Work out the finished part from the listing and answer in its coordinate system (mm). A direction names the side the tool comes from. Coordinates: 2 decimals unless noted, no trailing zeros. Loops run counter-clockwise (first coordinate to the right, second up) from the corner with the lowest first, then second, coordinate; pieces in that order, holes last. Notation, with made-up numbers: M -37.75,61 L -15.75,61 A4 ccw -15.75,66 Z; hole C 13,-35.5 d7. An arc over 180 degrees is marked long. Write each question's results on one line, items separated by ' | '.
Autodesk Fusion 360 part; units mm, degrees
sketch "Sketch1" plane through (0, 0, 0) normal (0, 0, 1) x (1, 0, 0)
  line L0 (0, 0) -> (139.7, 0)
  line L1 (139.7, 0) -> (139.7, 25)
  line L2 (139.7, 25) -> (0, 25)
  line L3 (0, 25) -> (0, 0)
  dimension "d1" = 139.7
  dimension "d2" = 25
extrude "Extrude1" add sketch "Sketch1" along normal blind 5
sketch "Sketch2" plane through (0, 0, 0) normal (0, 0, 1) x (1, 0, 0)
  point P0 (6.35, 12.5)
  point P1 (133.35, 12.5)
hole "Hole1" at (6.35, 12.5, 0) at (133.35, 12.5, 0) direction (0, 0, 1) diameter 5.5 depth 13 tip angle 118 counterbore diameter 9.1 counterbore depth 1
sketch "Sketch4" plane through (0, 0, 0) normal (0, 0, -1) x (1, 0, 0)
  circle A0 centre (6.35, -12.5) radius 4.55
  circle A1 centre (133.35, -12.5) radius 4.55
  line L0 (0, 0) -> (0, -25)
  line L1 (0, -25) -> (139.7, -25)
  line L2 (139.7, -25) -> (139.7, 0)
  line L3 (139.7, 0) -> (0, 0)
  point P0 (49.85, -12.5)
  point P1 (89.85, -12.5)
hole "Hole3" at (89.85, 12.5, 0) at (49.85, 12.5, 0) direction (0, 0, 1) diameter 5.5 depth 13 tip angle 118
1) Which of the six approach directions +Z, -Z, +X, -X, +Y, -Y give full straight-line access (tool end or side, diameter ignored) to faces 4 (the face through (139.7, 12, 2)), 5 (the face through (9.3, 12.4, 1))?
Check result:
face 4: +Z, -Z, +X, +Y, -Y | face 5: -Z
2) Straight lines are drawn through the part: probe 1 along X at (y, z) = (12.75, 3.4); probe 2 along X at (y, z) = (12.5, 0.7); probe 3 along Y at (x, z) = (133.35, 0.3). For each, find the intervals that lie inside material, in ascending order. Write a range as [from, to].
Check result:
probe 1: [0, 3.61], [9.09, 47.11], [52.59, 87.11], [92.59, 130.61], [136.09, 139.7] | probe 2: [0, 1.8], [10.9, 47.1], [52.6, 87.1], [92.6, 128.8], [137.9, 139.7] | probe 3: [0, 7.95], [17.05, 25]
3) Find section A-A, the plane x = 6.35. Give the vertices of the cut face in (y, z), and give its area (3 significant figures).
Check result:
outline: M 0,0 L 7.95,0 L 7.95,1 L 9.75,1 L 9.75,5 L 0,5 Z; M 15.25,1 L 17.05,1 L 17.05,0 L 25,0 L 25,5 L 15.25,5 Z | area: 93.9 mm^2
4) Find section D-D, the plane y = 13.25. Give the vertices of the cut face in (x, z), and give its area (3 significant figures).
Check result:
outline: M 0,0 L 1.86,0 L 1.86,1 L 3.7,1 L 3.7,5 L 0,5 Z; M 9,1 L 10.84,1 L 10.84,0 L 47.2,0 L 47.2,5 L 9,5 Z; M 52.5,0 L 87.2,0 L 87.2,5 L 52.5,5 Z; M 92.5,0 L 128.86,0 L 128.86,1 L 130.7,1 L 130.7,5 L 92.5,5 Z; M 136,1 L 137.84,1 L 137.84,0 L 139.7,0 L 139.7,5 L 136,5 Z | area: 585 mm^2
5) For a pull along X with two mould halves and no side action, classify faces 1 (the face through (0, 13, 2)), 2 (the face through (130.623, 12.142, 3.028)), 3 (the face through (69, 13, 0)) as released by +X, released by -X, zero draft, split by the parting line, or undercut.
Check result:
face 1: released by -X | face 2: undercut | face 3: zero draft
6) Find section C-C, the plane x = 89.85. Give the vertices of the cut face in (y, z).
Check result:
outline: M 0,0 L 9.75,0 L 9.75,5 L 0,5 Z; M 15.25,0 L 25,0 L 25,5 L 15.25,5 Z
7) Given pin 1 Ø7 at (x, y) = (133.35, 12.5) entering from -Z; pin 2 Ø4.5 at (x, y) = (6.35, 12.5) entering from +Z, each flat-ended and moving along its own axis, determine where each tip first touches the part or whether it passes through.
Check result:
pin 1: z = 1 | pin 2: through
8) Find section B-B, the plane z = 2.8. Give the vertices of the cut face in (x, y), and give its area (3 significant figures).
Check result:
outline: M 0,0 L 139.7,0 L 139.7,25 L 0,25 Z; hole C 6.35,12.5 d5.5; hole C 49.85,12.5 d5.5; hole C 89.85,12.5 d5.5; hole C 133.35,12.5 d5.5 | area: 3,400 mm^2
